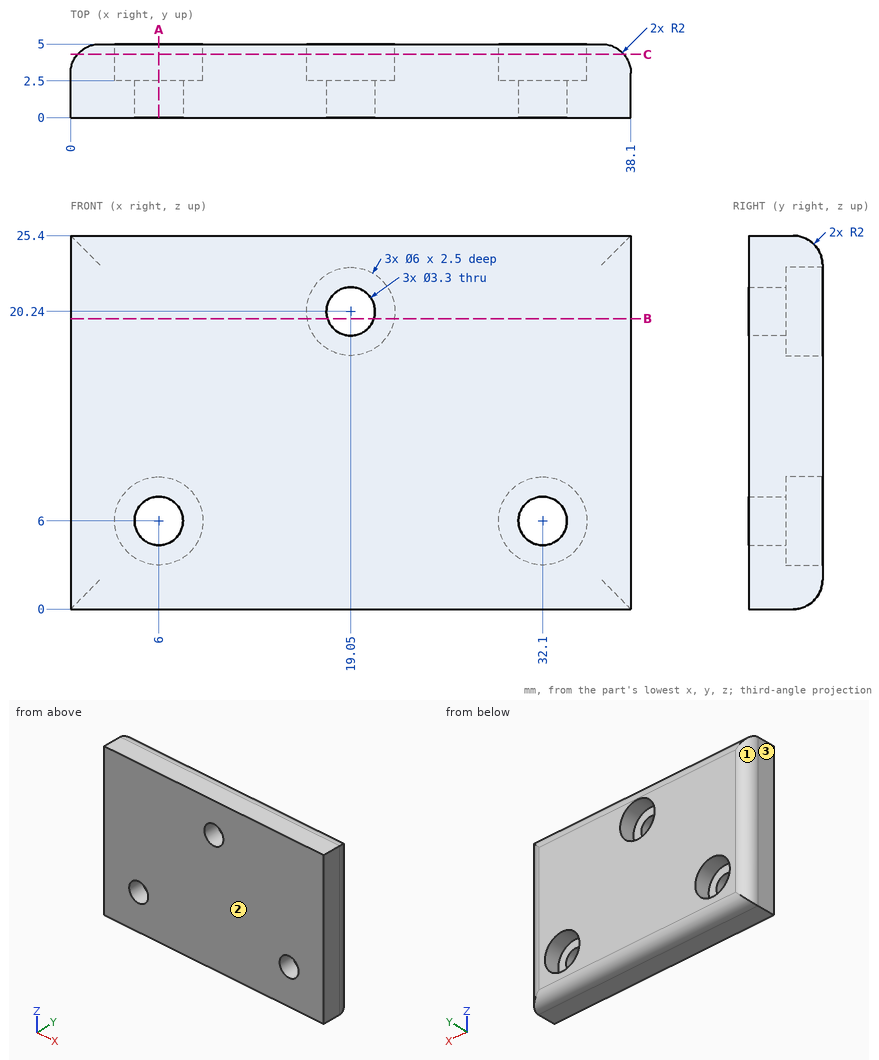
Drawing for the job (mm, zero at the part's lowest x, y, z). Round coordinates to 2 decimals unless told otherwise and drop trailing zeros. Loops run counter-clockwise (first coordinate to the right, second up) from the corner with the lowest first, then second, coordinate; pieces in that order, holes last.
1. Drop flat-ended pins along their axis: P1, Ø3.5, axis at x = 6, z = 6, coming from the +Y side; P2, Ø1.5, axis at y = 4, z = 7.5, coming from the -X side. Give the stop position or say it passes through.
Check values:
P1: stops at y = 2.5
P2: stops at x = 0.02
2. Band-saw the part on A-A, the plane x = 6. List the corners of the cut face in (y, z), and give its area (3 significant figures).
Check values:
outline: (0, 0) - (3, 0) arc R2 ccw to (5, 2) - (5, 3) - (2.5, 3) - (2.5, 4.35) - (0, 4.35) - close; (0, 7.65) - (2.5, 7.65) - (2.5, 9) - (5, 9) - (5, 23.4) arc R2 ccw to (3, 25.4) - (0, 25.4) - close
area: 102 mm2
3. Wall check: probe 1 along X at (y, z) = (1.35, 6); probe 2 along X at (y, z) = (4, 6); probe 3 along Z at (x, y) = (19.05, 1.3). Give the ranges that are in metal, low to high.
Check values:
probe 1: x = 0 to 4.35, 7.65 to 30.45, 33.75 to 38.1
probe 2: x = 0.27 to 3, 9 to 29.1, 35.1 to 37.83
probe 3: z = 0 to 18.59, 21.89 to 25.4
4. Band-saw the part on C-C, the plane y = 4.3. List the corners of the cut face in (x, z), and give its area (3 significant figures).
Check values:
outline: (0.48, 0.48) - (37.62, 0.48) - (37.62, 24.92) - (0.48, 24.92) - close; hole circle Ø6 at (6, 6); hole circle Ø6 at (19.05, 20.24); hole circle Ø6 at (32.1, 6)
area: 823 mm2
5. Band-saw the part on B-B, the plane z = 19.75. List the corners of the cut face in (x, y).
Check values:
outline: (0, 0) - (17.47, 0) - (17.47, 2.5) - (16.09, 2.5) - (16.09, 5) - (2, 5) arc R2 ccw to (0, 3) - close; (20.63, 0) - (38.1, 0) - (38.1, 3) arc R2 ccw to (36.1, 5) - (22.01, 5) - (22.01, 2.5) - (20.63, 2.5) - close
6. Mould opens along Y. For the marked faces 1, 2 and 3 say: +Y half, -Y half, draft (parallel to the pull), parting line (faces both ways), or undercut.
Check values:
face 1: +Y half
face 2: -Y half
face 3: draft
